from build123d import *

# Parameters (mm, degrees)
PAD_DEPTH              = 3
SKETCH001_W            = 18.3
SKETCH001_H            = 18.1
POCKET_DEPTH           = 3.001
LINEARPATTERN_COUNT    = 4
LINEARPATTERN_PITCH    = 35
HOLE_D                 = 3.4
HOLE_CBORE_D           = 5.8
HOLE_CBORE_DEPTH       = 1.5
SKETCH004_W            = 22.3
SKETCH004_H            = 22.1
SKETCH004_W_2          = 18.3
SKETCH004_H_2          = 18.1
PAD001_DEPTH           = 2
LINEARPATTERN001_COUNT = 4
LINEARPATTERN001_PITCH = 35
FILLET_R               = 1
FILLET001_R            = 1
FILLET002_R            = 1


with BuildPart() as part:
    # Sketch → Pad (new body)
    with BuildSketch(Plane.XY):
        with BuildLine():
            Line((145, 49), (0, 49))
            Line((0, 49), (0, 0))
            Line((0, 0), (155, 0))
            Line((155, 0), (155, 39))
            ThreePointArc((155, 39), (152.071068, 46.071068), (145, 49))
        make_face()
    extrude(amount=PAD_DEPTH)

    # Sketch001 (on Face7 of Pad) → Pocket (cut, through all)
    with BuildSketch(Plane.XY.offset(3)):
        with Locations((25.15, 34.05)):
            Rectangle(SKETCH001_W, SKETCH001_H)
    pocket = extrude(amount=-POCKET_DEPTH, mode=Mode.SUBTRACT)

    # LinearPattern: Pocket ×4
    with Locations(*[(i * LINEARPATTERN_PITCH, 0, 0) for i in range(1, LINEARPATTERN_COUNT)]):
        add(pocket, mode=Mode.SUBTRACT)

    # Hole (through all)
    with Locations(Plane.XY.offset(3)):
        with Locations((8, 25), (147, 25)):
            CounterBoreHole(HOLE_D / 2, HOLE_CBORE_D / 2, HOLE_CBORE_DEPTH)

    # Sketch004 (on Face4 of Hole) → Pad001 (join)
    with BuildSketch(Plane(origin=(0, 0, 0), x_dir=(1, 0, 0), z_dir=(0, 0, -1))):
        with Locations((25.15, -34.05)):
            Rectangle(SKETCH004_W, SKETCH004_H)
        with Locations((25.15, -34.05)):
            Rectangle(SKETCH004_W_2, SKETCH004_H_2, mode=Mode.SUBTRACT)
    pad001 = extrude(amount=PAD001_DEPTH)

    # LinearPattern001: Pad001 ×4
    with Locations(*[(i * LINEARPATTERN001_PITCH, 0, 0) for i in range(1, LINEARPATTERN001_COUNT)]):
        add(pad001)

    # Fillet
    fillet_edges = [part.edges().sort_by_distance(p)[0] for p in [
        (72.5, 49, 3),
    ]]
    fillet(fillet_edges, radius=FILLET_R)

    # Fillet001
    fillet001_edges = [part.edges().sort_by_distance(p)[0] for p in [
        (77, 0, 3),
    ]]
    fillet(fillet001_edges, radius=FILLET001_R)

    # Fillet002
    fillet002_edges = [part.edges().sort_by_distance(p)[0] for p in [
        (0, 24.5, 3),
    ]]
    fillet(fillet002_edges, radius=FILLET002_R)


solid = part.part
Check sheet for the modelled part. Datum: model origin and axes. Units: mm. A direction names the side the tool comes from. Give positions to 0.01 mm unless a question says otherwise; leave off trailing zeros. Write each loop counter-clockwise with the first axis right and the second up, starting at its lowest first coordinate (ties: lowest second). Pieces come first, ordered by that corner, then holes. Notation, with made-up numbers: (47.5, -30) -> (67.5, -30) arc R28 cw to (67.5, -7) -> close; hole circle Ø11 at (44, 19). An arc over 180 degrees is marked (long way). One line per item, written item: value. Start each with the question number.
Item 1: Draft check along Y on faces 4 (the flat face through (130, 25, 1)), 5 (the cylindrical face through (152.15, 45.99, 0.99)), 6 (the flat face through (76, 25, 3)). Enter one of: +Y half, -Y half, draft (parallel to the pull), parting line (faces both ways), or undercut.
Item 2: Gauge pin test, flat ends, axial feed: pin 1 (1.6 mm diameter, centred on y = 30.5, z = -1, fed in from -X); pin 2 (1 mm diameter, centred on y = 31.5, z = -1, fed in from +X); pin 3 (2 mm diameter, centred on x = 91, z = -1.5, fed in from -Y). Record the tip position at first contact, or that the pin passes through.
Item 3: Section check C-C on y = 10. Record the cut outline in (x, z), then the cut area to 3 significant figures.
Item 4: Tool access check on faces 1 (the flat face through (8, 23, 1.5)), 2 (the flat face through (60, 44, -2)), 3 (the flat face through (25, 25, 1)). Record the directions out of +Z, -Z, +X, -X, +Y, -Y that give a thin tool (end or side, any length) a straight path to the whole face; none if there is none.
Item 5: Section check A-A on x = 20. Record the cut outline in (y, z).
Item 6: Section check B-B on y = 35.5. State how many separate pieces and enclosed holes the cut face has, then the cut area to 3 significant figures.
Item 7: Material ranges on probe 1 along X at (y, z) = (23, 1.95); probe 2 along Y at (x, z) = (99, 0.35); probe 3 along X at (y, z) = (12.5, 2.05), recorded low to high. Write a range as from..to.
Results list:
1. face 4: undercut
1. face 5: +Y half
1. face 6: draft
2. pin 1: x = 14
2. pin 2: x = 141.3
2. pin 3: y = 23
3. outline: (0, 0) -> (155, 0) -> (155, 2) arc R1 ccw to (154, 3) -> (1, 3) arc R1 ccw to (0, 2) -> close
3. area: 465 mm²
4. face 1: +Z
4. face 2: -Z, +X, -X, +Y, -Y
4. face 3: +Z, -Z
5. outline: (0, 0) -> (23, 0) -> (23, -2) -> (25, -2) -> (25, 3) -> (1, 3) arc R1 ccw to (0, 2) -> close; (43.1, -2) -> (45.1, -2) -> (45.1, 0) -> (49, 0) -> (49, 2) arc R1 ccw to (48, 3) -> (43.1, 3) -> close
6. separate pieces: 5
6. enclosed holes: 0
6. area: 277 mm²
7. probe 1: 0..5.9, 10.1..144.9, 149.1..155
7. probe 2: 0..25, 43.1..49
7. probe 3: 0..155
